Geometry check sheet. Reference: the model listing, model coordinates, mm. Coordinates: 2 decimals unless noted, no trailing zeros. Loops run counter-clockwise (first coordinate to the right, second up) from the corner with the lowest first, then second, coordinate; pieces in that order, holes last.
from build123d import *

# Parameters (mm, degrees)
F2_FACE_W = 36
F2_FACE_H = 4


with BuildPart() as f2:
    # F2: sweep along a path in F1
    with BuildLine(Plane.XY) as f2_path:
        Line((0, 0), (-36, 0))
    # F0 (on Right) → F2 (sweep)
    with BuildSketch(Plane.YZ):
        with BuildLine():
            ThreePointArc((12, 0), (0, -12), (-12, 0))
            Line((-12, 0), (-16, 0))
            ThreePointArc((-16, 0), (0, -15.9386387537), (16, 0))
            Line((16, 0), (12, 0))
        make_face()
    sweep(path=f2_path.line)

    # F2_face (on face) → F5 section 0
    with BuildSketch(Plane(origin=(-18, -14, 0), x_dir=(1, 0, 0), z_dir=(0, 0, 1))):
        Rectangle(F2_FACE_W, F2_FACE_H)
    # F4 (on offset) → F5 section 1
    with BuildSketch(Plane.XY.offset(12)):
        with BuildLine():
            ThreePointArc((0, -25.5), (-17.9775042284, -26.8098477779), (-36, -26.5))
            Line((-36, -26.5), (-36, -32.5))
            Line((-36, -32.5), (0, -32.5))
            Line((0, -32.5), (0, -25.5))
        make_face()
    loft()


solid = f2.part
(1) Sectioned sample at B-B on y = 0. Record the cut outline in (x, z).
Findings:
outline: (-36, -15.94) - (0, -15.94) - (0, -12) - (-36, -12) - close
(2) Draft check along Y on faces 1 (the flat face through (-18, 14, 0)), 2 (the cylindrical face through (-18, 0, -12)), 3 (the flat face through (-18.252, -24.365, 6.084)). Enter one of: +Y half, -Y half, draft (parallel to the pull), parting line (faces both ways), or undercut.
Findings:
face 1: draft
face 2: undercut
face 3: -Y half
(3) Sectioned sample at A-A on z = -0.75. Record the cut outline in (x, y), and give its area (3 significant figures).
Findings:
outline: (-36, -15.98) - (0, -15.98) - (0, -11.98) - (-36, -11.98) - close; (-36, 11.98) - (0, 11.98) - (0, 15.98) - (-36, 15.98) - close
area: 288 mm2
(4) Sectioned sample at C-C on y = -9. Record the cut outline in (x, z).
Findings:
outline: (-36, -13.17) - (0, -13.17) - (0, -7.94) - (-36, -7.94) - close
(5) Gauge pin test, flat ends, axial feed: pin 1 Ø1 at (x, y) = (-12.5, -9.5) entering from +Z; pin 2 Ø1 at (x, z) = (-23, 8) entering from -Y; pin 3 Ø3 at (x, y) = (-8, -23.5) entering from +Z; pin 4 Ø4 at (y, z) = (10, -3.5) entering from -X. Record the tip position at first contact, or that the pin passes through.
Findings:
pin 1: stops at z = -6.63
pin 2: stops at y = -27.69
pin 3: stops at z = 10.92
pin 4: stops at x = -36
(6) Scan lines: L1, parallel to Y at x = -11, z = -2.5; L2, parallel to Y at x = -8.5, z = -9.5; L3, parallel to Z at x = -32, y = -20.5. Record each from-to range of solid material in increasing order.
Findings:
L1: y = -15.79 to -11.74, 11.74 to 15.79
L2: y = -12.83 to -7.33, 7.33 to 12.83
L3: z = 3.27 to 6.93
